```python
from build123d import *

# Parameters (mm, degrees)
SKETCH1_R           = 15.875
BOSS_EXTRUDE1_DEPTH = 25.4
CUT_EXTRUDE1_DEPTH  = 26.4


with BuildPart() as part:
    # Sketch1 → Boss-Extrude1 (new body)
    with BuildSketch(Plane(origin=(0, 0, 0), x_dir=(1, 0, 0), z_dir=(0, 1, 0))):
        Circle(SKETCH1_R)
    extrude(amount=BOSS_EXTRUDE1_DEPTH)

    # Sketch2 → Cut-Extrude1 (cut, through all)
    with BuildSketch(Plane(origin=(0, 25.4, 0), x_dir=(1, 0, 0), z_dir=(0, 1, 0))):
        Polygon((-6.35, 0), (-5.616765158, 1.27), (-12.7, 1.27), (-12.7, -1.27), (-5.616765158, -1.27), align=None)
        Polygon((3.175, -5.499261314), (5.616765158, -1.27), (-5.616765158, -1.27), (-3.175, -5.499261314), align=None)
        Polygon((6.35, 0), (5.616765158, 1.27), (-5.616765158, 1.27), (-6.35, 0), (-5.616765158, -1.27), (5.616765158, -1.27), align=None)
        Polygon((5.616765158, 1.27), (3.175, 5.499261314), (-3.175, 5.499261314), (-5.616765158, 1.27), align=None)
        Polygon((12.7, 1.27), (5.616765158, 1.27), (6.35, 0), (5.616765158, -1.27), (12.7, -1.27), align=None)
    extrude(amount=-CUT_EXTRUDE1_DEPTH, mode=Mode.SUBTRACT)


solid = part.part
```
The model under review builds one solid part; all positions refer to its coordinate system, in mm. A direction names the side the tool comes from. Round coordinates to 2 decimals unless told otherwise and drop trailing zeros. Write each loop counter-clockwise with the first axis right and the second up, starting at its lowest first coordinate (ties: lowest second). Pieces come first, ordered by that corner, then holes. Notation, with made-up numbers: (77, -31) -> (117, -31) arc R20 ccw to (117, 1) -> close; hole circle Ø7 at (20, 43). An arc over 180 degrees is marked (long way). Use CSV: the item, a comma, the result in double quotes.
Q1. To check wall thickness, follow probe 1 along Z at (x, y) = (10.5, 16.5); probe 2 along Z at (x, y) = (10, 23); probe 3 along X at (y, z) = (20.25, -4.5). State the ranges of each line that lie inside material, in increasing order. Write a range as [from, to].
Checks:
probe 1,"[-11.91, -1.27], [1.27, 11.91]"
probe 2,"[-12.33, -1.27], [1.27, 12.33]"
probe 3,"[-15.22, -3.75], [3.75, 15.22]"
Q2. Consider section B-B (y = 6). Give the boundary of the cut face in (x, z) (3 decimals).
Checks:
outline,"circle Ø31.75 at (0, 0); hole (-12.7, -1.27) -> (-5.617, -1.27) -> (-3.175, -5.499) -> (3.175, -5.499) -> (5.617, -1.27) -> (12.7, -1.27) -> (12.7, 1.27) -> (5.617, 1.27) -> (3.175, 5.499) -> (-3.175, 5.499) -> (-5.617, 1.27) -> (-12.7, 1.27) -> close"
Q3. For pin 1 Ø5 at (y, z) = (17, 10) entering from -X; pin 2 Ø3.5 at (x, y) = (-7.5, 15) entering from +Z; pin 3 Ø2 at (y, z) = (18, -9) entering from +X, all flat-tipped, find the tip position at first contact; note any pin that passes through.
Checks:
pin 1,"x = -13.99"
pin 2,"z = 14.8"
pin 3,"x = 13.71"
Q4. Consider section D-D (z = -12). Give the boundary of the cut face in (x, y), then the cut area to 3 significant figures.
Checks:
outline,"(-10.39, 0) -> (10.39, 0) -> (10.39, 25.4) -> (-10.39, 25.4) -> close"
area,"528 mm²"
Q5. Mouldability with a two-part tool opening along Z and no side actions: class faces 1 (the flat face through (9, 13, -1.27)), 2 (the flat face through (0, 0, 7)), 3 (the cylindrical face through (-3.441, 12.522, 15.497)) as released by +Z, released by -Z, zero draft, split by the parting line, or undercut.
Checks:
face 1,"undercut"
face 2,"zero draft"
face 3,"split by the parting line"
Q6. Consider section A-A (x = 0). Give the boundary of the cut face in (y, z) (3 decimals).
Checks:
outline,"(0, -15.875) -> (25.4, -15.875) -> (25.4, -5.499) -> (0, -5.499) -> close; (0, 5.499) -> (25.4, 5.499) -> (25.4, 15.875) -> (0, 15.875) -> close"
Q7. Consider section C-C (z = 0). Give the boundary of the cut face in (x, y) (3 decimals), then the cut area to 3 significant figures.
Checks:
outline,"(-15.875, 0) -> (-12.7, 0) -> (-12.7, 25.4) -> (-15.875, 25.4) -> close; (12.7, 0) -> (15.875, 0) -> (15.875, 25.4) -> (12.7, 25.4) -> close"
area,"161 mm²"
Q8. For faces 4 (the flat face through (0, 25.4, 7)), 5 (the flat face through (-4.41, 12.88, 3.36)), list the 3-axis set-ups (+Z, -Z, +X, -X, +Y, -Y) from which the entire face can be reached by the end or side of a thin tool; tool diameter is ignored.
Checks:
face 4,"+Z, -Z, +X, -X, +Y"
face 5,"+Y, -Y"
